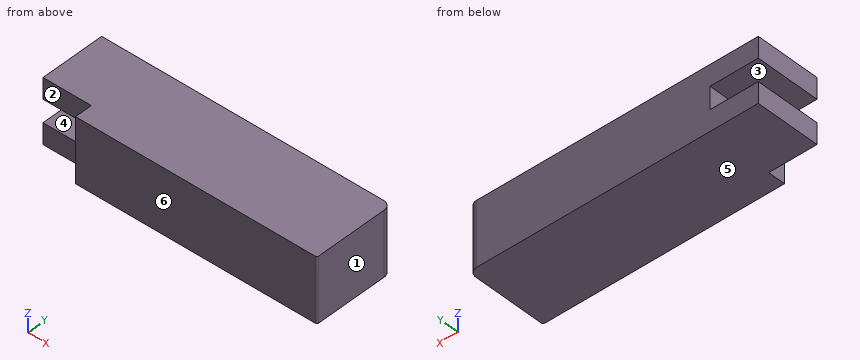
from build123d import *

# Parameters (mm, degrees)
EXTRUDE_1_DEPTH     = 20
SKETCH_2_W          = 30
SKETCH_2_H          = 40
CUT_EXTRUDE_1_DEPTH = 7
FILLET_1_R          = 5
FILLET_2_R          = 1


with BuildPart() as part:
    # 스케치1 → 보스-돌출1 (new, symmetric)
    with BuildSketch(Plane.XY):
        Polygon((0, -40), (30, -40), (30, -50.78), (180, -50.78), (180, 0), (0, 0), align=None)
    extrude(amount=EXTRUDE_1_DEPTH, both=True)

    # 스케치2 → 컷-돌출1 (cut, symmetric)
    with BuildSketch(Plane.XY):
        with Locations((15, -20)):
            Rectangle(SKETCH_2_W, SKETCH_2_H)
    extrude(amount=CUT_EXTRUDE_1_DEPTH, both=True, mode=Mode.SUBTRACT)

    # 필렛1
    fillet_1_edges = [part.edges().sort_by_distance(p)[0] for p in [
        (180, 0, 0),
    ]]
    fillet(fillet_1_edges, radius=FILLET_1_R)

    # 필렛2
    fillet_2_edges = [part.edges().sort_by_distance(p)[0] for p in [
        (180, -50.78, 0),
    ]]
    fillet(fillet_2_edges, radius=FILLET_2_R)


solid = part.part
Geometry: final body of the model. Coordinates: model frame, mm. Face numbers are marked on the shaded views. A direction names the side the tool comes from. Round coordinates to 2 decimals unless told otherwise and drop trailing zeros. Order: outer loops, then holes, each group sorted by start corner. A loop starts at its lowest first (then second) coordinate and runs counter-clockwise, first axis right, second up. Notation, with made-up numbers: (1, -36.5) -> (7, -36.5) arc R21 cw to (7, -5.5) -> close; hole circle Ø1 at (-29, -18.5). An arc over 180 degrees is marked (long way). Put each result on its own line as item: value. Start each with the question number.
Q1. Section C-C on z = 2. Return the cut outline in (x, y).
Q2. Line query: probe 1 along Z at (x, y) = (15.5, -11.5); probe 2 along X at (y, z) = (-43, -7.5); probe 3 along Y at (x, z) = (27, 14). Output: solid intervals per line, ascending.
Q3. Reachability of the marked faces 1 and 2 from +Z, -Z, +X, -X, +Y, -Y: full face, straight path, thin tool, end or side. Return the list, or none.
Q4. Section A-A on z = -16. Return the cut outline in (x, y).
Q5. Pull-direction query (Z, two-part tool) for the marked faces 3, 4, 5 and 6; classes: +Z half, -Z half, draft (parallel to the pull), parting line (faces both ways), or undercut.
Q6. First-contact query: pin 1 (14.5 mm diameter, centred on x = 12, z = -14, fed in from -Y). Flat tip, straight axial feed; report the tip coordinate or a pass-through.
Q7. Section B-B on y = -12. Return the cut outline in (x, z).
Ans:
1. outline: (30, -50.78) -> (179, -50.78) arc R1 ccw to (180, -49.78) -> (180, -5) arc R5 ccw to (175, 0) -> (30, 0) -> close
2. probe 1: z = -20 to -7, 7 to 20
2. probe 2: x = 30 to 180
2. probe 3: y = -40 to 0
3. face 1: +Z, -Z, +X, +Y, -Y
3. face 2: +Z, -Z, -X, -Y
4. outline: (0, -40) -> (30, -40) -> (30, -50.78) -> (179, -50.78) arc R1 ccw to (180, -49.78) -> (180, -5) arc R5 ccw to (175, 0) -> (0, 0) -> close
5. face 3: undercut
5. face 4: undercut
5. face 5: -Z half
5. face 6: draft
6. pin 1: stops at y = -40
7. outline: (0, -20) -> (180, -20) -> (180, 20) -> (0, 20) -> (0, 7) -> (30, 7) -> (30, -7) -> (0, -7) -> close
